Model file for the job. Use its own axes, mm. A direction names the side the tool comes from. Coordinates: 2 decimals unless noted, no trailing zeros. Order: outer loops, then holes, each group sorted by start corner. A loop starts at its lowest first (then second) coordinate and runs counter-clockwise, first axis right, second up.
from build123d import *

# Parameters (mm, degrees)
SKETCH1_W           = 35
SKETCH1_H           = 30
SKETCH1_R           = 1.7
BOSS_EXTRUDE1_DEPTH = 2.5
SKETCH3_W           = 18
SKETCH3_H           = 5
CUT_EXTRUDE1_DEPTH  = 5
SKETCH4_W           = 2.551904925
SKETCH4_H           = 30
BOSS_EXTRUDE2_DEPTH = 1.75
SKETCH5_W           = 2.448095075
SKETCH5_H           = 30
SKETCH5_W_2         = 2.551904925
SKETCH5_W_3         = 5
BOSS_EXTRUDE3_DEPTH = 1
SKETCH6_W           = 35
SKETCH6_H           = 5.25
BOSS_EXTRUDE4_DEPTH = 1


with BuildPart() as part:
    # Sketch1 → Boss-Extrude1 (new body)
    with BuildSketch(Plane.XY):
        with Locations((17.5, 15)):
            Rectangle(SKETCH1_W, SKETCH1_H)
        with Locations((5.5, 27)):
            Circle(SKETCH1_R, mode=Mode.SUBTRACT)
        with Locations((29.5, 27)):
            Circle(SKETCH1_R, mode=Mode.SUBTRACT)
        with Locations((29.5, 3)):
            Circle(SKETCH1_R, mode=Mode.SUBTRACT)
        with Locations((5.5, 3)):
            Circle(SKETCH1_R, mode=Mode.SUBTRACT)
    extrude(amount=BOSS_EXTRUDE1_DEPTH)

    # Sketch3 → Cut-Extrude1 (cut)
    with BuildSketch(Plane.XY.offset(2.5)):
        with Locations((17.5, 2.5)):
            Rectangle(SKETCH3_W, SKETCH3_H)
    extrude(amount=-CUT_EXTRUDE1_DEPTH, mode=Mode.SUBTRACT)

    # Sketch4 → Boss-Extrude2 (add)
    with BuildSketch(Plane.XY.offset(2.5)):
        with Locations((1.275952463, 15)):
            Rectangle(SKETCH4_W, SKETCH4_H)
        with Locations((33.724047537, 15)):
            Rectangle(SKETCH4_W, SKETCH4_H)
    extrude(amount=BOSS_EXTRUDE2_DEPTH)

    # Sketch5 → Boss-Extrude3 (add)
    with BuildSketch(Plane.XY.offset(4.25)):
        with Locations((3.775952463, 15)):
            Rectangle(SKETCH5_W, SKETCH5_H)
        with Locations((1.275952463, 15)):
            Rectangle(SKETCH5_W_2, SKETCH5_H)
        with Locations((32.5, 15)):
            Rectangle(SKETCH5_W_3, SKETCH5_H)
    extrude(amount=BOSS_EXTRUDE3_DEPTH)

    # Sketch6 → Boss-Extrude4 (add)
    with BuildSketch(Plane(origin=(0, 30, 0), x_dir=(1, 0, 0), z_dir=(0, 1, 0))):
        with Locations((17.5, -2.625)):
            Rectangle(SKETCH6_W, SKETCH6_H)
    extrude(amount=BOSS_EXTRUDE4_DEPTH)


solid = part.part
Q1. Cut at D-D, the plane y = 3. List the corners of the cut face in (x, z).
Established:
outline: (0, 0) - (3.8, 0) - (3.8, 2.5) - (2.55, 2.5) - (2.55, 4.25) - (5, 4.25) - (5, 5.25) - (0, 5.25) - close; (7.2, 0) - (8.5, 0) - (8.5, 2.5) - (7.2, 2.5) - close; (26.5, 0) - (27.8, 0) - (27.8, 2.5) - (26.5, 2.5) - close; (30, 4.25) - (32.45, 4.25) - (32.45, 2.5) - (31.2, 2.5) - (31.2, 0) - (35, 0) - (35, 5.25) - (30, 5.25) - close
Q2. Mould opens along X. For faces 6 (the face through (0, 15, 3)), 7 (the face through (4, 15, 4.25)), 8 (the face through (26.5, 2, 1)), 9 (the face through (17, 31, 3)) say: pulls with the +X half, pulls with the -X half, needs draft (parallel to the pull), parting line crosses it, or undercut.
Established:
face 6: pulls with the -X half
face 7: undercut
face 8: undercut
face 9: needs draft
Q3. Cut at C-C, the plane z = 1.7. List the corners of the cut face in (x, y).
Established:
outline: (0, 0) - (8.5, 0) - (8.5, 5) - (26.5, 5) - (26.5, 0) - (35, 0) - (35, 31) - (0, 31) - close; hole circle Ø3.4 at (5.5, 3); hole circle Ø3.4 at (5.5, 27); hole circle Ø3.4 at (29.5, 3); hole circle Ø3.4 at (29.5, 27)
Q4. Drop flat-ended pins along their axis: P1, Ø0.8, axis at x = 22, z = 4, coming from the -Y side; P2, Ø9, axis at x = 19.5, y = 12, coming from the +Z side; P3, Ø2, axis at x = 19.5, z = 1, coming from the -Y side. Give the stop position or say it passes through.
Established:
P1: stops at y = 30
P2: stops at z = 2.5
P3: stops at y = 5
Q5. Probe line 1 (Y direction, x = 29.5, z = 1.75); line 2 (X direction, y = 27.5, z = 5.05); line 3 (X direction, y = 1, z = 1.9). List the from-to ranges inside material, lowest first.
Established:
line 1: y = 0 to 1.3, 4.7 to 25.3, 28.7 to 31
line 2: x = 0 to 5, 30 to 35
line 3: x = 0 to 8.5, 26.5 to 35
Q6. Which spindle directions (+Z, -Z, +X, -X, +Y, -Y) get a long thin tool onto all of the face, cutting with end or side? Do faces 1 (the face through (17, 19, 0)), 2 (the face through (8.5, 2, 1)), 3 (the face through (32.448, 15, 3)), 4 (the face through (5.279, 28.686, 1.232)), 5 (the face through (30, 15, 5)). Say none if no direction does.
Established:
face 1: -Z, +X, -X, +Y, -Y
face 2: +Z, -Z, -Y
face 3: -Y
face 4: -Z
face 5: +Z, -Y
Q7. Cut at A-A, the plane x = 29.5. List the corners of the cut face in (y, z), plus the area to 4 significant figures.
Established:
outline: (0, 0) - (1.3, 0) - (1.3, 2.5) - (0, 2.5) - close; (4.7, 0) - (25.3, 0) - (25.3, 2.5) - (4.7, 2.5) - close; (28.7, 0) - (31, 0) - (31, 5.25) - (30, 5.25) - (30, 2.5) - (28.7, 2.5) - close
area: 63.25 mm2
Q8. Cut at B-B, the plane y = 27. List the corners of the cut face in (x, z), plus the area to 3 significant figures.
Established:
outline: (0, 0) - (3.8, 0) - (3.8, 2.5) - (2.55, 2.5) - (2.55, 4.25) - (5, 4.25) - (5, 5.25) - (0, 5.25) - close; (7.2, 0) - (27.8, 0) - (27.8, 2.5) - (7.2, 2.5) - close; (30, 4.25) - (32.45, 4.25) - (32.45, 2.5) - (31.2, 2.5) - (31.2, 0) - (35, 0) - (35, 5.25) - (30, 5.25) - close
area: 89.4 mm2
